from build123d import *

# Parameters (mm, degrees)
BOSS_EXTRUDE1_DEPTH = 1.6
SKETCH2_R           = 1.6
CUT_EXTRUDE1_DEPTH  = 22.279332696
FILLET1_R           = 1
CUT_EXTRUDE2_DEPTH  = 22.279332696
LPATTERN1_COUNT     = 3
LPATTERN1_PITCH     = 6
LPATTERN1_COL_COUNT = 3
LPATTERN1_COL_PITCH = 6


with BuildPart() as part:
    # Sketch1 → Boss-Extrude1 (new body)
    with BuildSketch(Plane(origin=(0, 0, 0), x_dir=(1, 0, 0), z_dir=(0, 1, 0))):
        Polygon((3.5, 2), (7.5, 2), (7.5, -2), (17.5, -2), (17.5, -12), (-17.5, -12), (-17.5, -2), (-7.5, -2), (-7.5, 2), (-3.5, 2), (-3.5, 5.5), (3.5, 5.5), align=None)
    extrude(amount=BOSS_EXTRUDE1_DEPTH)

    # Sketch2 → Cut-Extrude1 (cut, through all)
    with BuildSketch(Plane(origin=(0, 1.6, 0), x_dir=(1, 0, 0), z_dir=(0, 1, 0))):
        with Locations(Location((0, 2, 0), (0, 0, 270))):
            Circle(SKETCH2_R)
    extrude(amount=-CUT_EXTRUDE1_DEPTH, mode=Mode.SUBTRACT)

    # Fillet1
    fillet1_edges = [part.edges().sort_by_distance(p)[0] for p in [
        (7.5, 0.8, 2),
        (17.5, 0.8, 2),
        (17.5, 0.8, 12),
        (-17.5, 0.8, 12),
        (-17.5, 0.8, 2),
        (-7.5, 0.8, 2),
        (-7.5, 0.8, -2),
        (-3.5, 0.8, -2),
        (-3.5, 0.8, -5.5),
        (3.5, 0.8, -5.5),
        (3.5, 0.8, -2),
        (7.5, 0.8, -2),
    ]]
    fillet(fillet1_edges, radius=FILLET1_R)

    # Sketch3 → Cut-Extrude2 (cut, through all)
    with BuildSketch(Plane(origin=(0, 1.6, 0), x_dir=(1, 0, 0), z_dir=(0, 1, 0))):
        with BuildLine():
            Line((-1.2, -9.5), (-1.2, -4.5))
            ThreePointArc((-1.2, -4.5), (0, -3.3), (1.2, -4.5))
            Line((1.2, -4.5), (1.2, -9.5))
            ThreePointArc((1.2, -9.5), (0, -10.7), (-1.2, -9.5))
        make_face()
    cut_extrude2 = extrude(amount=-CUT_EXTRUDE2_DEPTH, mode=Mode.SUBTRACT)

    # LPattern1: Cut-Extrude2 ×3
    with Locations(*[(i * LPATTERN1_PITCH, 0, 0) for i in range(1, LPATTERN1_COUNT)]):
        add(cut_extrude2, mode=Mode.SUBTRACT)

    # LPattern1 col: Cut-Extrude2 ×3
    with Locations(*[(-i * LPATTERN1_COL_PITCH, 0, 0) for i in range(1, LPATTERN1_COL_COUNT)]):
        add(cut_extrude2, mode=Mode.SUBTRACT)


solid = part.part
Part model, mm, in its own coordinate system. A direction names the side the tool comes from. Give positions to 0.01 mm unless a question says otherwise; leave off trailing zeros. Loops run counter-clockwise (first coordinate to the right, second up) from the corner with the lowest first, then second, coordinate; pieces in that order, holes last. Notation, with made-up numbers: M 19.5,-1.75 L 27.5,-1.75 A22 cw 27.5,8.25 Z; hole C -2.5,59.5 d6. An arc over 180 degrees is marked long. Put each result on its own line as item: value. Start each with the question number.
1) Saw through at B-B (z = 9). List the corners of the cut face in (x, y).
2) Probe probe 1 along X at (y, z) = (1.4, 5.25); probe 2 along Z at (x, y) = (-12, 1.5); probe 3 along X at (y, z) = (1.3, 10.25). List the from-to ranges inside material, lowest first.
3) 3-axis set-ups, long thin cutter, end or side, ignore diameter. For faces 5 (the flat face through (-7.2, 1, 7)), 6 (the flat face through (-13, 1, 2)), 7 (the flat face through (12, 1, 2)): which of +Z, -Z, +X, -X, +Y, -Y reach the whole face in a straight line?
4) Saw through at C-C (x = 0.5). List the corners of the cut face in (y, z), then the cut area to 3 significant figures.
5) Saw through at A-A (x = -6). List the corners of the cut face in (y, z).
6) Saw through at D-D (x = -12). List the corners of the cut face in (y, z), then the cut area to 3 significant figures.
7) Flat gauge pins, fed straight in: pin 1 (5 mm diameter, centred on x = -8, z = -2.5, fed in from -Y); pin 2 (0.5 mm diameter, centred on y = 1, z = 0, fed in from +X); pin 3 (3 mm diameter, centred on x = 0, z = -2, fed in from -Y); pin 4 (0.5 mm diameter, centred on y = 1, z = 0, fed in from -X). Where does each tip first touch, or does it go through?
8) Pull direction X, two halves, no side cores. Call faces 1 (the flat face through (0, 0, 3)), 2 (the flat face through (10.8, 1, 7)), 3 (the cylindrical face through (0, 0.8, 3.3)), 4 (the flat face through (17.5, 1, 7)): +X half, -X half, draft (parallel to the pull), parting line (faces both ways), or undercut.
Numbers:
1. outline: M -17.5,0 L -13.2,0 L -13.2,1.6 L -17.5,1.6 Z; M -10.8,0 L -7.2,0 L -7.2,1.6 L -10.8,1.6 Z; M -4.8,0 L -1.2,0 L -1.2,1.6 L -4.8,1.6 Z; M 1.2,0 L 4.8,0 L 4.8,1.6 L 1.2,1.6 Z; M 7.2,0 L 10.8,0 L 10.8,1.6 L 7.2,1.6 Z; M 13.2,0 L 17.5,0 L 17.5,1.6 L 13.2,1.6 Z
2. probe 1: -17.5 to -13.2, -10.8 to -7.2, -4.8 to -1.2, 1.2 to 4.8, 7.2 to 10.8, 13.2 to 17.5
2. probe 2: 2 to 3.3, 10.7 to 12
2. probe 3: -17.5 to -12.94, -11.06 to -6.94, -5.06 to -0.94, 0.94 to 5.06, 6.94 to 11.06, 12.94 to 17.5
3. face 5: +Y, -Y
3. face 6: -Z, -X, +Y, -Y
3. face 7: -Z, +X, +Y, -Y
4. outline: M 0,-5.5 L 1.6,-5.5 L 1.6,-3.52 L 0,-3.52 Z; M 0,-0.48 L 1.6,-0.48 L 1.6,3.41 L 0,3.41 Z; M 0,10.59 L 1.6,10.59 L 1.6,12 L 0,12 Z
4. area: 11.6 mm^2
5. outline: M 0,-2 L 1.6,-2 L 1.6,3.3 L 0,3.3 Z; M 0,10.7 L 1.6,10.7 L 1.6,12 L 0,12 Z
6. outline: M 0,2 L 1.6,2 L 1.6,3.3 L 0,3.3 Z; M 0,10.7 L 1.6,10.7 L 1.6,12 L 0,12 Z
6. area: 4.16 mm^2
7. pin 1: y = 0
7. pin 2: x = 7.5
7. pin 3: through
7. pin 4: x = -7.5
8. face 1: draft
8. face 2: undercut
8. face 3: undercut
8. face 4: +X half
